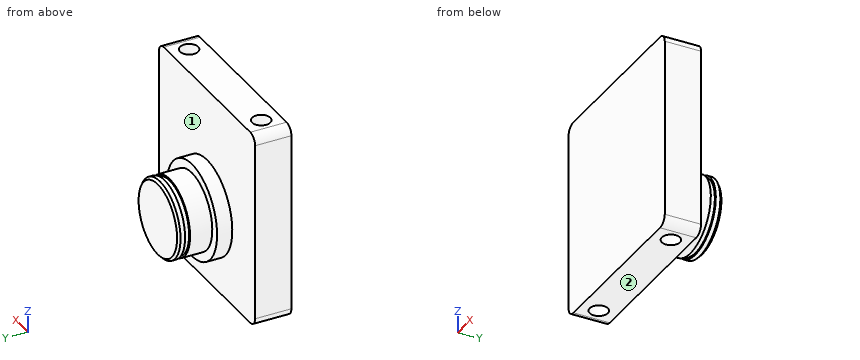
```python
from build123d import *

# Parameters (mm, degrees)
SKETCH_1_W          = 40
SKETCH_1_H          = 43.5
EXTRUDE_1_DEPTH     = 8
SKETCH_2_R          = 10.5
EXTRUDE_2_DEPTH     = 3.35
SKETCH_3_R          = 8.5
EXTRUDE_3_DEPTH     = 7.5
SKETCH_4_R          = 2
CUT_EXTRUDE_1_DEPTH = 52.454567339
CUT_EXTRUDE_START   = -1.1
SKETCH_5_R          = 8.5
SKETCH_5_R_2        = 8.1
CUT_EXTRUDE_2_DEPTH = 1.1
CHAMFER_1_SIZE      = 0.5
FILLET_1_R          = 2


with BuildPart() as part:
    # 草图1 → 凸台-拉伸1 (new body)
    with BuildSketch(Plane(origin=(0, 0, 0), x_dir=(1, 0, 0), z_dir=(0, 1, 0))):
        with Locations((0, -4.75)):
            Rectangle(SKETCH_1_W, SKETCH_1_H)
    extrude(amount=EXTRUDE_1_DEPTH)

    # 草图2 → 凸台-拉伸2 (add)
    with BuildSketch(Plane(origin=(0, 8, 0), x_dir=(1, 0, 0), z_dir=(0, 1, 0))):
        with Locations(Location((0, 0, 0), (0, 0, 270))):
            Circle(SKETCH_2_R)
    extrude(amount=EXTRUDE_2_DEPTH)

    # 草图3 → 凸台-拉伸3 (add)
    with BuildSketch(Plane(origin=(0, 11.35, 0), x_dir=(1, 0, 0), z_dir=(0, 1, 0))):
        with Locations(Location((0, 0, 0), (0, 0, 270))):
            Circle(SKETCH_3_R)
    extrude(amount=EXTRUDE_3_DEPTH)

    # 草图4 → 切除-拉伸1 (cut, through all)
    with BuildSketch(Plane(origin=(0, 0, -17), x_dir=(-1, 0, 0), z_dir=(0, 0, -1))):
        with Locations((-15, 4)):
            Circle(SKETCH_4_R)
        with Locations((15, 4)):
            Circle(SKETCH_4_R)
    extrude(amount=-CUT_EXTRUDE_1_DEPTH, mode=Mode.SUBTRACT)

    # 草图5 → 切除-拉伸2 (cut)
    with BuildSketch(Plane(origin=(0, 17.35, 0), x_dir=(1, 0, 0), z_dir=(0, 1, 0)).offset(CUT_EXTRUDE_START)):
        with Locations(Location((0, 0, 0), (0, 0, 270))):
            Circle(SKETCH_5_R)
        with Locations(Location((0, 0, 0), (0, 0, 270))):
            Circle(SKETCH_5_R_2, mode=Mode.SUBTRACT)
    extrude(amount=CUT_EXTRUDE_2_DEPTH, mode=Mode.SUBTRACT)

    # 倒角1
    chamfer_1_edges = [part.edges().sort_by_distance(p)[0] for p in [
        (0, 18.85, -8.5),
    ]]
    chamfer(chamfer_1_edges, length=CHAMFER_1_SIZE)

    # 圆角1
    fillet_1_edges = [part.edges().sort_by_distance(p)[0] for p in [
        (20, 4, 26.5),
        (-20, 4, 26.5),
        (-20, 4, -17),
        (20, 4, -17),
    ]]
    fillet(fillet_1_edges, radius=FILLET_1_R)


solid = part.part
```
The model under review builds one solid part; all positions refer to its coordinate system, in mm. Face numbers are marked on the shaded views. A direction names the side the tool comes from. Round coordinates to 2 decimals unless told otherwise and drop trailing zeros. Loops run counter-clockwise (first coordinate to the right, second up) from the corner with the lowest first, then second, coordinate; pieces in that order, holes last. Notation, with made-up numbers: M -6.5,70 L 34.5,70 A16 ccw 34.5,99 Z; hole C 64.5,33 d8. An arc over 180 degrees is marked long. Write item = value, one per line.
Item 1: For line 1 (Y direction, x = 15, z = 0.5); line 2 (X direction, y = 2.75, z = -6.5); line 3 (X direction, y = 4.5, z = 18), list the stretches that pass through material, from the lowest coordinate up. Write a range as [from, to].
Return value:
line_1 = [0, 2], [6, 8]
line_2 = [-20, -16.56], [-13.44, 13.44], [16.56, 20]
line_3 = [-20, -16.94], [-13.06, 13.06], [16.94, 20]
Item 2: Take a section at D-D on x = 0. Write out the cut boundary in (y, z), then the cut area to 3 significant figures.
Return value:
outline = M 0,-17 L 8,-17 L 8,-10.5 L 11.35,-10.5 L 11.35,-8.5 L 16.25,-8.5 L 16.25,-8.1 L 17.35,-8.1 L 17.35,-8.5 L 18.35,-8.5 L 18.85,-8 L 18.85,8 L 18.35,8.5 L 17.35,8.5 L 17.35,8.1 L 16.25,8.1 L 16.25,8.5 L 11.35,8.5 L 11.35,10.5 L 8,10.5 L 8,26.5 L 0,26.5 Z
area = 545 mm2
Item 3: Take a section at B-B on x = -15. Write out the cut boundary in (y, z).
Return value:
outline = M 0,-17 L 2,-17 L 2,26.5 L 0,26.5 Z; M 6,-17 L 8,-17 L 8,26.5 L 6,26.5 Z
Item 4: Take a section at C-C on y = 4. Write out the cut boundary in (x, z).
Return value:
outline = M -20,-15 A2 ccw -18,-17 L -17,-17 L -17,26.5 L -18,26.5 A2 ccw -20,24.5 Z; M -13,-17 L 13,-17 L 13,26.5 L -13,26.5 Z; M 17,-17 L 18,-17 A2 ccw 20,-15 L 20,24.5 A2 ccw 18,26.5 L 17,26.5 Z
Item 5: Take a section at A-A on z = 0. Write out the cut boundary in (x, y), then the cut area to 3 significant figures.
Return value:
outline = M -20,0 L 20,0 L 20,8 L 10.5,8 L 10.5,11.35 L 8.5,11.35 L 8.5,16.25 L 8.1,16.25 L 8.1,17.35 L 8.5,17.35 L 8.5,18.35 L 8,18.85 L -8,18.85 L -8.5,18.35 L -8.5,17.35 L -8.1,17.35 L -8.1,16.25 L -8.5,16.25 L -8.5,11.35 L -10.5,11.35 L -10.5,8 L -20,8 Z; hole C -15,4 d4; hole C 15,4 d4
area = 492 mm2
Item 6: Machinability: for the marked faces 1 and 2, which of the approach directions +Z, -Z, +X, -X, +Y, -Y give a long, thin tool a straight path to every point of the face, cutting with its end or side? Answer none if there is none.
Return value:
face_1 = +Y
face_2 = -Z, +X, -X, +Y, -Y
Item 7: Insertion check: P1, Ø8, axis at x = 9.5, z = -8, coming from the +Y side; P2, Ø8, axis at x = 13, z = 13.5, coming from the +Y side; P3, Ø5, axis at x = 5, y = 11.5, coming from the +Z side. Each pin has a flat end and moves straight along its axis. Give the tip position at first contact, or say it passes through.
Return value:
P1 = 18.43
P2 = 8
P3 = 10.2
